Verification items for this drawing (mm, ordinates from the low corner). A direction names the side the tool comes from. Give positions to 0.01 mm unless a question says otherwise; leave off trailing zeros. Write each loop counter-clockwise with the first axis right and the second up, starting at its lowest first coordinate (ties: lowest second). Pieces come first, ordered by that corner, then holes. Notation, with made-up numbers: (-30.5, -24.75) -> (-15.5, -24.75) arc R35 ccw to (-15.5, 7.25) -> close; hole circle Ø10 at (-31.75, -34). An arc over 180 degrees is marked (long way). Answer as a JSON object with one key per item and string values.
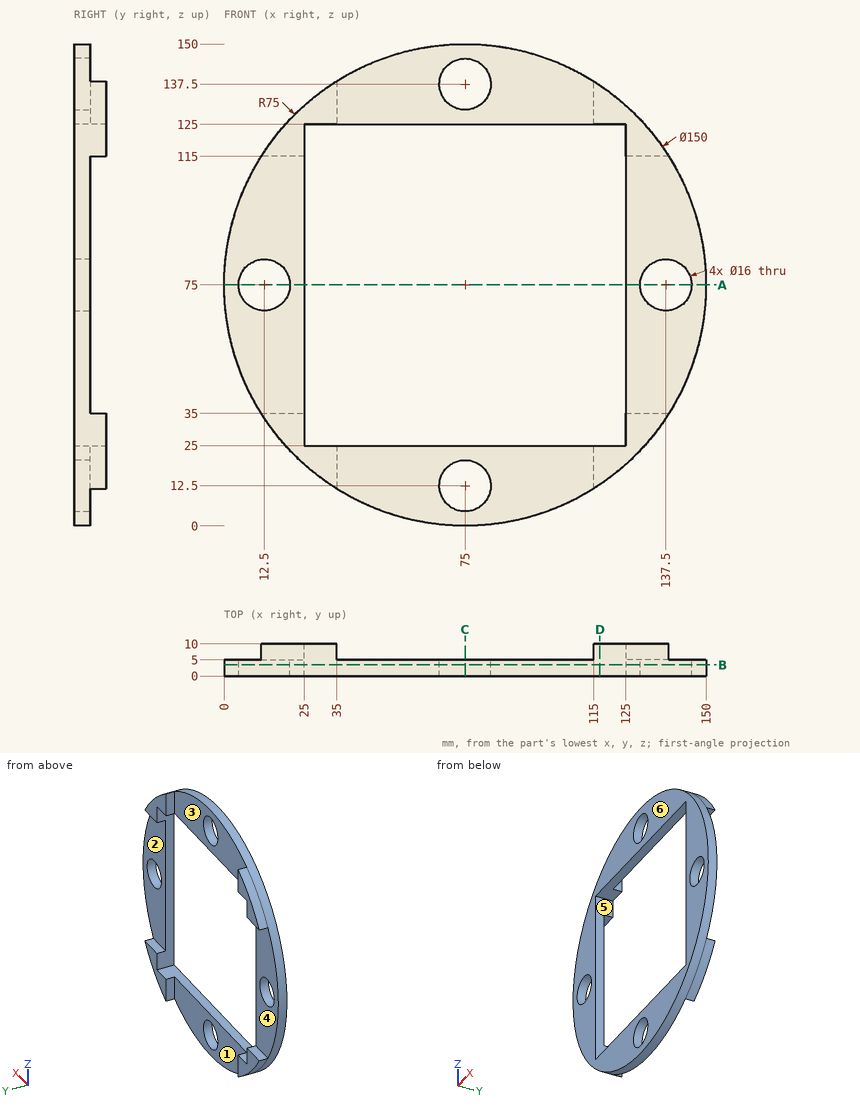
1. Scan lines: L1, parallel to X at y = 2.95, z = 75; L2, parallel to Y at x = 51.5, z = 126.5; L3, parallel to X at y = 3.25, z = 139. Record each from-to range of solid material in increasing order. Write a range as [from, to].
Determined:
{"L1": "[0, 4.5], [20.5, 25], [125, 129.5], [145.5, 150]", "L2": "[0, 5]", "L3": "[35.9, 67.14], [82.86, 114.1]"}
2. Access from +Z, -Z, +X, -X, +Y, -Y to the whole of each face (thin tool, end or side, straight path). Record for the marked faces 4, 5 and 6.
Determined:
{"face 4": "+X, -X, +Y", "face 5": "+Y, -Y", "face 6": "+Z, -Z, +X, -X, -Y"}
3. Mould release check, pull along X, two halves, no side actions. Record for the marked faces 1, 2 and 3: released by +X, released by -X, zero draft, split by the parting line, or undercut.
Determined:
{"face 1": "undercut", "face 2": "zero draft", "face 3": "undercut"}
4. Sectioned sample at D-D, the plane x = 117. Enter the section's corners in (y, z).
Determined:
{"outline": "(0, 12.86) -> (10, 12.86) -> (10, 25) -> (0, 25) -> close; (0, 125) -> (10, 125) -> (10, 137.14) -> (0, 137.14) -> close"}
5. Sectioned sample at C-C, the plane x = 75. Enter the section's corners in (y, z).
Determined:
{"outline": "(0, 0) -> (5, 0) -> (5, 4.5) -> (0, 4.5) -> close; (0, 20.5) -> (5, 20.5) -> (5, 25) -> (0, 25) -> close; (0, 125) -> (5, 125) -> (5, 129.5) -> (0, 129.5) -> close; (0, 145.5) -> (5, 145.5) -> (5, 150) -> (0, 150) -> close"}
6. Go/stop test with flat-tipped pins: P1, Ø6, axis at x = 69, y = 6.5, coming from the -Z side; P2, Ø1.5, axis at y = 7, z = 130, coming from the -X side; P3, Ø2.5, axis at x = 17.5, y = 7.5, coming from the -Z side. Record where each tip stops, or that it passes through.
Determined:
{"P1": "z = 0.08", "P2": "x = 23.21", "P3": "z = 25.39"}
7. Sectioned sample at B-B, the plane y = 3.5. Enter the section's corners in (x, z).
Determined:
{"outline": "circle Ø150 at (75, 75); hole circle Ø16 at (12.5, 75); hole (25, 25) -> (125, 25) -> (125, 125) -> (25, 125) -> close; hole circle Ø16 at (75, 12.5); hole circle Ø16 at (75, 137.5); hole circle Ø16 at (137.5, 75)"}
8. Sectioned sample at A-A, the plane z = 75. Enter the section's corners in (x, y).
Determined:
{"outline": "(0, 0) -> (4.5, 0) -> (4.5, 5) -> (0, 5) -> close; (20.5, 0) -> (25, 0) -> (25, 5) -> (20.5, 5) -> close; (125, 0) -> (129.5, 0) -> (129.5, 5) -> (125, 5) -> close; (145.5, 0) -> (150, 0) -> (150, 5) -> (145.5, 5) -> close"}
